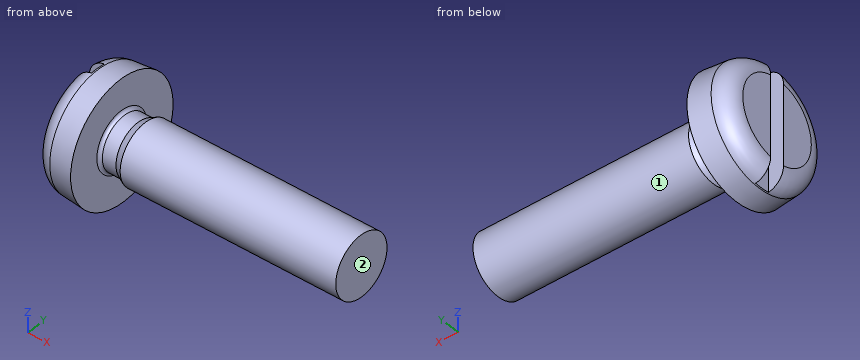
Autodesk Inventor part; units mm, degrees
ref_plane "Work Plane1" through (30.1625, 0, 0) normal (0, 0, -1) x (1, 0, 0)
ref_plane "YZ Plane" through (0, 0, 0) normal (1, 0, 0) x (0, 1, 0)
ref_plane "XZ Plane" through (0, 0, 0) normal (0, 1, 0) x (-1, 0, 0)
sketch "Эскиз1" plane through (0, 0, 0) normal (0, 0, 1) x (1, 0, 0)
  line L0 (-1.3, 0) -> (8, 0)
  line L1 (8, 0) -> (8, 1)
  line L2 (8, 1) -> (0.8, 1)
  line L3 (0.8, 1) -> (0.5545, 0.8772)
  line L4 (0.5545, 0.8772) -> (0, 0.8772)
  line L5 (0, 0.8772) -> (0, 2)
  line L6 (-3.16, 0) -> (9.86, 0)
  line L7 (0, -0.4) -> (0, 2.4)
  line L8 (-1.3, 0) -> (-1.3, 1.8863)
  line L9 (0, 2) -> (-1.3, 1.8863)
  line L10 (0.8, 1) -> (0, 1) construction
  dimension "d0" = 8
  dimension "d1" = 7.2
  dimension "d2" = 0.2455
  dimension "d3" = 1.3
  dimension "d4" = 2
  dimension "d5" = 1.7545
  dimension "d9" = 4
  dimension "d10" = 5
revolve "Базовый элемент" add sketch "Эскиз1" angle 360 about axis through (-1.3, 0, 0) along (1, 0, 0)
sketch "Эскиз2" plane through (-1.3, 0, 0) normal (-1, 0, 0) x (0, 0, 1)
  circle A0 centre (0, 0) radius 2
  line L0 (0, 0) -> (0, 1.8863)
  line L1 (-2, 0.25) -> (2, 0.25)
  line L2 (2, 0.25) -> (2, -0.25)
  line L3 (2, -0.25) -> (-2, -0.25)
  line L4 (-2, -0.25) -> (-2, 0.25)
  line L5 (-2, 0) -> (2, 0) construction
  line L6 (0, 0.25) -> (0, -0.25) construction
  dimension "d11" = 0.5
  dimension "d12" = 4
fillet "Сопряжение1" radius 0.6 1 edges at (-1.3, -1.8863, 0)
extrude "Паз" cut sketch "Эскиз2" against normal blind 0.5 contours A0 L3 L1 | L2 L3 A0 | A0 L1 L2 | A0 L4 L1 | L3 L4 A0
thread "Резьба"
ref_plane "Work Plane1" through (30.1625, 0, 0) normal (0, 0, -1) x (1, 0, 0)
fillet "Fillet5" radius 0.1 1 edges at (0, -0.8772, 0)
equation "\"d11\" = SBR"
equation "\"d12\" = KOD"
equation "\"d19\" = STI"
equation "\"d41\" = R"
equation "\"d14\" = RR"
equation "\"d15\" = GEL"
equation "\"d0\" = NLG"
equation "\"d1\" = GEL"
equation "\"d3\" = KOH"
equation "\"d4\" = GD"
equation "\"d5\" = BDM"
equation "\"d9\" = KOD"
equation "\"d10\" = KEWI"
equation "\"GD\" = NND"
equation "\"NLG\" = 8"
equation "\"GEL\" = 7.2"
equation "\"KOD\" = 4"
equation "\"KOH\" = 1.3"
equation "\"GAL\" = 0.61345 * PTC"
equation "\"R\" = 0.1"
equation "\"BDM\" = 1.7545"
equation "\"GUL\" = 0.61345 * PTC"
equation "\"RR\" = 0.6"
equation "\"SBR\" = 0.5"
equation "\"STI\" = 0.5"
equation "\"KEWI\" = 5deg"
equation "\"PTC\" = 0.4"
equation "\"THREADDIA\" = 2"
equation "\"TOA\" = 30deg"
equation "\"NND\" = 2"
equation "\"GD1\" = THREADDIA - 1.2269 * PTC"
properties part number "ISO 1580 - M2 x 8" material "Сталь, мягкая"
Could you check a few things on this model? Use its own coordinates, in mm. Face numbers are marked on the shaded views. A direction names the side the tool comes from. Give positions to 0.01 mm unless a question says otherwise; leave off trailing zeros. Loops run counter-clockwise (first coordinate to the right, second up) from the corner with the lowest first, then second, coordinate; pieces in that order, holes last. Notation, with made-up numbers: M 3,85.5 L 7,85.5 A18 cw 7,115.5 Z; hole C 75,81.5 d8. An arc over 180 degrees is marked long. Answer as a JSON object with one key per item and string values.
Q1. If I drill on probe 1 along X at (y, z) = (-0.05, 0.6); probe 2 along X at (y, z) = (-0.9, -1.05); probe 3 along Z at (x, y) = (-0.25, 0.4), over which ranges is the centre line in solid material (lowest first)? Write a range as [from, to].
Values found:
{"probe 1": "x = [-0.8, 8]", "probe 2": "x = [-1.3, 0]", "probe 3": "z = [-1.94, 1.94]"}
Q2. Suppose I cut it at C-C, the plane x = 6.5. List the corners of the cut face in (y, z) for me, plus the area to 3 significant figures.
Values found:
{"outline": "C 0,0 d2", "area": "3.14 mm²"}
Q3. Suppose I cut it at B-B, the plane z = 0. List the corners of the cut face in (x, y) for me, plus the area to 3 significant figures.
Values found:
{"outline": "M -1.3,-1.34 A0.6 ccw -0.75,-1.93 L 0,-2 L 0,-0.98 A0.1 cw 0.1,-0.88 L 0.55,-0.88 L 0.8,-1 L 8,-1 L 8,1 L 0.8,1 L 0.55,0.88 L 0.1,0.88 A0.1 cw 0,0.98 L 0,2 L -0.75,1.93 A0.6 ccw -1.3,1.34 L -1.3,0.25 L -0.8,0.25 L -0.8,-0.25 L -1.3,-0.25 Z", "area": "20.5 mm²"}
Q4. For P1, Ø1, axis at x = 2.5, y = -1, coming from the -Z side; P2, Ø1.5, axis at x = 6, z = -1, coming from the +Y side, each with a flat end and sliding along its axis, tell me the tip position at first contact or that it passes through.
Values found:
{"P1": "stops at z = -0.87", "P2": "stops at y = 0.97"}
Q5. Suppose I cut it at A-A, the plane y = 0. List the corners of the cut face in (x, z) for me, plus the area to 3 significant figures.
Values found:
{"outline": "M -0.8,-1.93 A0.6 ccw -0.75,-1.93 L 0,-2 L 0,-0.98 A0.1 cw 0.1,-0.88 L 0.55,-0.88 L 0.8,-1 L 8,-1 L 8,1 L 0.8,1 L 0.55,0.88 L 0.1,0.88 A0.1 cw 0,0.98 L 0,2 L -0.75,1.93 A0.6 ccw -0.8,1.93 Z", "area": "19.0 mm²"}
Q6. For the marked faces 1 and 2, which set-ups out of +Z, -Z, +X, -X, +Y, -Y let a thin tool reach every point of the face, with its end or its side?
Values found:
{"face 1": "+X", "face 2": "+Z, -Z, +X, +Y, -Y"}
